Autodesk Inventor part; units mm, degrees
ref_plane "MSC_PT1" through (5.1, 0, 0) normal (1, 0, 0) x (0, 1, 0)
ref_plane "MSC_PT2" through (0, 0, 0) normal (-1, 0, 0) x (0, -1, 0)
ref_plane "MSC_PF1" through (0, 0, 0) normal (1, 0, 0) x (0, 1, 0)
sketch "Sketch1" plane through (0, 0, 0) normal (1, 0, 0) x (0, 1, 0)
  line L0 (4, 2.3094) -> (4, -2.3094)
  line L1 (4, -2.3094) -> (0, -4.6188)
  line L2 (0, -4.6188) -> (-4, -2.3094)
  line L3 (-4, -2.3094) -> (-4, 2.3094)
  line L4 (-4, 2.3094) -> (0, 4.6188)
  line L5 (0, 4.6188) -> (4, 2.3094)
  circle A0 centre (0, 0) radius 4 construction
  dimension "d0" = 8
extrude "Extrusion1" add sketch "Sketch1" along normal blind 5.1
sketch "Sketch2" plane through (5.1, 0, 0) normal (1, 0, 0) x (0, 1, 0)
  line L0 (-4, 2.3094) -> (0, 4.6188)
  line L1 (0, -4.6188) -> (-4, -2.3094)
  line L2 (-4, 2.3094) -> (4, -2.3094) construction
  line L3 (-4, -2.3094) -> (4, 2.3094) construction
  point P0 (0, 0)
hole "Hole1" at (5.1, 0, 0) direction (-1, 0, 0) diameter 4.134 end through all
chamfer "Chamfer1" distance 0.4 angle 45 2 edges at (5.1, 0, 2.067) (0, 0, 2.067)
sketch "Sketch3" plane through (0, 0, 0) normal (0, 1, 0) x (-1, 0, 0)
  line L0 (-7.0172, 0) -> (2.1698, 0)
  line L1 (-5.7048, 0) -> (0.8574, 0)
  line L2 (-5.1, 0) -> (-5.1, -4.6188)
  line L3 (-5.1, -4.6188) -> (0, -4.6188)
  line L4 (0, -4.6188) -> (0, 0)
  line L5 (-5.1, -2.3094) -> (-5.1, -4.6188)
  line L6 (0, -2.3094) -> (0, -4.6188)
  line L7 (0, -4.6188) -> (-5.1, -4.6188)
  line L8 (-5.1, -4) -> (-4.7427, -4.6188)
  line L9 (-5.1, -4.6188) -> (-5.1, -4)
  line L10 (-5.1, -4.6188) -> (-4.7427, -4.6188)
  line L11 (0, -4) -> (-0.3573, -4.6188)
  line L12 (-0.3573, -4.6188) -> (0, -4.6188)
  line L13 (0, -4.6188) -> (0, -4)
  dimension "d32" = 4
  dimension "d33" = 30
revolve "Revolution1" cut sketch "Sketch3" angle 360 about axis through (0, 0, 0) along (-1, 0, 0) contours L8 L3 L2 | L4 L3 L11
ref_plane "MSC_PT1" through (5.1, 0, 0) normal (1, 0, 0) x (0, 1, 0)
ref_plane "MSC_PT2" through (0, 0, 0) normal (-1, 0, 0) x (0, -1, 0)
ref_plane "MSC_PF1" through (0, 0, 0) normal (1, 0, 0) x (0, 1, 0)
equation "\"d0\" = Smax"
equation "\"d1\" = Mmax"
equation "\"d10\" = 0.5 * PTC"
equation "\"d32\" = 0.5 * Smax"
equation "\"NND\" = 5"
equation "\"Smax\" = 8"
equation "\"Mmax\" = 5.1"
equation "\"PTC\" = 0.8"
equation "\"THREADDIA\" = NND"
equation "\"TEMPLATE\" = 1.2345"
properties part number "ANSI B18.2.4.2M - M5x0.8" material "Steel, Mild"
Source: CAD feature listing. Evaluate the final solid. Frame: model axes, mm. Round coordinates to 2 decimals unless told otherwise and drop trailing zeros. Loops run counter-clockwise (first coordinate to the right, second up) from the corner with the lowest first, then second, coordinate; pieces in that order, holes last.
1. Section query A-A on x = 3.8. Output: boundary loops of the cut face in (y, z), and give its area (3 significant figures).
2. Mould query, pull axis Z, two halves, no side actions, for faces 1 (the cylindrical face through (2.52, 1.26, 1.64)), 2 (the flat face through (0, 2, 2)), 3 (the conical face through (0.087, 3.589, -2.084)), 4 (the flat face through (2.514, -2.028, 3.448)). Classes: released by +Z, released by -Z, zero draft, split by the parting line, or undercut.
3. Ray query, L1, parallel to Y at x = 2.05, z = 0; L2, parallel to Y at x = 3.3, z = -1; L3, parallel to Z at x = 2.25, y = -1.25. Return the intervals inside material, ascending.
4. Contact query for a flat-ended pin moving along its axis: pin 1 (1 mm diameter, centred on x = 2, y = 2.5, fed in from +Z). Output: stop coordinate, or through.
Answers below:
1. outline: (-4, -2.31) - (0, -4.62) - (4, -2.31) - (4, 2.31) - (0, 4.62) - (-4, 2.31) - close; hole circle Ø4.13 at (0, 0)
1. area: 42.0 mm2
2. face 1: undercut
2. face 2: zero draft
2. face 3: released by -Z
2. face 4: released by +Z
3. L1: y = -4 to -2.07, 2.07 to 4
3. L2: y = -4 to -1.81, 1.81 to 4
3. L3: z = -3.9 to -1.65, 1.65 to 3.9
4. pin 1: stops at z = 3.46
